```python
from build123d import *

# Parameters (mm, degrees)
SKETCH_1_W          = 85.5
SKETCH_1_H          = 23
SKETCH_1_W_2        = 3
SKETCH_1_H_2        = 18.5
SKETCH_1_W_3        = 70
SKETCH_1_H_3        = 12.711442786
EXTRUDE_1_DEPTH     = 19
SKETCH_2_W          = 85.5
SKETCH_2_H          = 23
EXTRUDE_2_DEPTH     = 2
SKETCH_3_R          = 2
CUT_EXTRUDE_1_DEPTH = 97


with BuildPart() as part:
    # 草圖1 → 填料-伸長1 (new body)
    with BuildSketch(Plane.XY):
        with Locations((-2.25, -0.25)):
            Rectangle(SKETCH_1_W, SKETCH_1_H)
        with Locations((36, 0)):
            Rectangle(SKETCH_1_W_2, SKETCH_1_H_2, mode=Mode.SUBTRACT)
        with Locations((-2.5, 0)):
            Rectangle(SKETCH_1_W_3, SKETCH_1_H_2, mode=Mode.SUBTRACT)
        with Locations((-40.5, 0)):
            Rectangle(SKETCH_1_W_2, SKETCH_1_H_3, mode=Mode.SUBTRACT)
    extrude(amount=EXTRUDE_1_DEPTH)

    # 草圖2 → 填料-伸長2 (add)
    with BuildSketch(Plane(origin=(0, 0, 0), x_dir=(-1, 0, 0), z_dir=(0, 0, -1))):
        with Locations((2.25, -0.25)):
            Rectangle(SKETCH_2_W, SKETCH_2_H)
    extrude(amount=EXTRUDE_2_DEPTH)

    # 草圖3 → 除料-伸長1 (cut)
    with BuildSketch(Plane(origin=(40.5, 0, 0), x_dir=(0, 0, -1), z_dir=(1, 0, 0))):
        with Locations(Location((-11, 0.282979523, 0), (0, 0, 90))):
            Circle(SKETCH_3_R)
    extrude(amount=-CUT_EXTRUDE_1_DEPTH, mode=Mode.SUBTRACT)


solid = part.part
```
Here's how the part is built. I have some questions about the finished solid (model axes, mm). A direction names the side the tool comes from. Give positions to 0.01 mm unless a question says otherwise; leave off trailing zeros. Loops run counter-clockwise (first coordinate to the right, second up) from the corner with the lowest first, then second, coordinate; pieces in that order, holes last. Notation, with made-up numbers: (20, 70.25) -> (61, 70.25) arc R22 cw to (61, 101.25) -> close; hole circle Ø9 at (13.5, -4.5). An arc over 180 degrees is marked (long way). Use one line per item in the form item = value. Start each with the question number.
1) Please list where these lines run through material, in increasing order: line 1 along X through (y, z) = (-5.75, 14.25); line 2 along X through (y, z) = (6.5, 12.25); line 3 along Y through (x, z) = (-9.5, 13.75).
2) Imagine slicing it at B-B (x = 10.5). Please give me the cut outline in (y, z), then the cut area to 4 significant figures.
3) Which directions (+Z, -Z, +X, -X, +Y, -Y) give clear straight access to the entire face, cutting with the end or side of a thin tool? Please do faces 1 (the face through (-3, -9.25, 9)), 2 (the face through (-2, -11.75, 9)).
4) Imagine slicing it at C-C (y = -4.75). Please give me the cut outline in (x, z), then the cut area to 4 significant figures.
5) Thinking about a two-plate mould opening in Y: for faces 3 (the face through (34.5, -2, 9)), 4 (the face through (40.5, -0.4, 8.6)), 5 (the face through (-2, 11.25, 9)), which applies, +Y half, -Y half, draft (parallel to the pull), parting line (faces both ways), or undercut?
6) Imagine slicing it at D-D (z = 7). Please give me the cut outline in (x, y).
7) For P1, Ø1.5, axis at x = -40, y = 1, coming from the +Z side; P2, Ø3, axis at y = 0.28, z = 11, coming from the +X side, each with a flat end and sliding along its axis, tell me the tip position at first contact or that it passes through.
Check values:
q1.line_1 = -45 to -42, -39 to -37.5, 32.5 to 34.5, 37.5 to 40.5
q1.line_2 = -45 to -37.5, 32.5 to 34.5, 37.5 to 40.5
q1.line_3 = -11.75 to -9.25, 9.25 to 11.25
q2.outline = (-11.75, -2) -> (11.25, -2) -> (11.25, 19) -> (9.25, 19) -> (9.25, 0) -> (-9.25, 0) -> (-9.25, 19) -> (-11.75, 19) -> close
q2.area = 131.5 mm^2
q3.face_1 = +Z
q3.face_2 = +Z, -Z, +X, -X, -Y
q4.outline = (-45, -2) -> (40.5, -2) -> (40.5, 19) -> (37.5, 19) -> (37.5, 0) -> (34.5, 0) -> (34.5, 19) -> (32.5, 19) -> (32.5, 0) -> (-37.5, 0) -> (-37.5, 19) -> (-39, 19) -> (-39, 0) -> (-42, 0) -> (-42, 19) -> (-45, 19) -> close
q4.area = 351.5 mm^2
q5.face_3 = undercut
q5.face_4 = draft
q5.face_5 = +Y half
q6.outline = (-45, -11.75) -> (40.5, -11.75) -> (40.5, 11.25) -> (-45, 11.25) -> close; hole (-42, -6.36) -> (-39, -6.36) -> (-39, 6.36) -> (-42, 6.36) -> close; hole (-37.5, -9.25) -> (32.5, -9.25) -> (32.5, 9.25) -> (-37.5, 9.25) -> close; hole (34.5, -9.25) -> (37.5, -9.25) -> (37.5, 9.25) -> (34.5, 9.25) -> close
q7.P1 = 0
q7.P2 = through
